Check sheet for the modelled part. Datum: model origin and axes. Units: mm. Face numbers are marked on the shaded views. A direction names the side the tool comes from. Round coordinates to 2 decimals unless told otherwise and drop trailing zeros. Write each loop counter-clockwise with the first axis right and the second up, starting at its lowest first coordinate (ties: lowest second). Pieces come first, ordered by that corner, then holes.
Item 1: Cross-section at D-D on x = 40. Enter the section's corners in (y, z).
Item 2: Cross-section at A-A on y = 15. Enter the section's corners in (x, z).
Item 3: Cross-section at B-B on y = -15.5. Enter the section's corners in (x, z), plus the area to 3 significant figures.
Item 4: Cross-section at C-C on z = 17. Enter the section's corners in (x, y), plus the area to 3 significant figures.
Item 5: Go/stop test with flat-tipped pins: pin 1 Ø8 at (x, y) = (12, 8.5) entering from +Z; pin 2 Ø1.5 at (y, z) = (4, -26) entering from -X; pin 3 Ø8 at (x, y) = (-34, 4.5) entering from -Z. Record where each tip stops, or that it passes through.
Item 6: Material ranges on line 1 (Z direction, x = -13.5, y = 5); line 2 (Z direction, x = 12, y = 14); line 3 (X direction, y = 9, z = -22), recorded low to high.
Item 7: Tool access check on the marked faces 1 and 2. Record the directions out of +Z, -Z, +X, -X, +Y, -Y that give a thin tool (end or side, any length) a straight path to the whole face; none if there is none.
Item 8: Release check for a two-part mould opening along Z. For the marked faces 3, 4 and 5 record: +Z half, -Z half, draft (parallel to the pull), parting line (faces both ways), or undercut.
from build123d import *

# Parameters (mm, degrees)
F1_DEPTH = 20
F2_DEPTH = 20


with BuildPart() as f1:
    # F0 (on Front) → F1 (new body, symmetric)
    with BuildSketch(Plane.XZ):
        Polygon((16.16565, -44.080839), (34.79936, -31.519093), (45.460955, -11.736702), (45.707994, 10.734426), (35.483882, 30.746426), (17.130841, 43.714791), (-5.14667, 46.668624), (-26.245141, 38.931237), (-41.331166, 22.275173), (-46.948719, 0.516136), (-41.810887, -21.361142), (-27.094684, -38.34484), (-6.171415, -46.544197), align=None)
        Polygon((21.260118, -15.324641), (11.703184, -23.449365), (-0.534809, -26.202123), (-12.650283, -22.952289), (-21.86773, -14.444363), (-26.075544, -2.627408), (-24.309764, 9.791456), (-16.974911, 19.967214), (-5.75131, 25.568725), (6.789846, 25.312748), (17.775531, 19.257927), (24.689056, 8.791346), (25.946615, -3.689226), align=None, mode=Mode.SUBTRACT)
    extrude(amount=F1_DEPTH, both=True)

    # F0 (on Front) → F2 (join)
    with BuildSketch(Plane.XZ):
        Polygon((-0.534809, -26.202123), (11.703184, -23.449365), (21.260118, -15.324641), (25.946615, -3.689226), (24.689056, 8.791346), (17.775531, 19.257927), (6.789846, 25.312748), (-5.75131, 25.568725), (-16.974911, 19.967214), (-24.309764, 9.791456), (-26.075544, -2.627408), (-21.86773, -14.444363), (-12.650283, -22.952289), align=None)
    extrude(amount=F2_DEPTH)


solid = f1.part
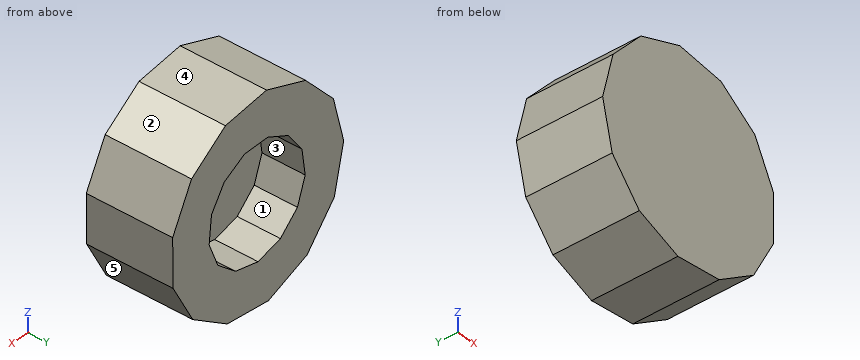
Response values:
1. outline: (-20, -21.87) - (20, -21.87) - (20, 21.91) - (-20, 21.91) - close
2. outline: (-46.95, 0.52) - (-41.81, -21.36) - (-27.09, -38.34) - (-6.17, -46.54) - (16.17, -44.08) - (34.8, -31.52) - (45.46, -11.74) - (45.71, 10.73) - (35.48, 30.75) - (17.13, 43.71) - (-5.15, 46.67) - (-26.25, 38.93) - (-41.33, 22.28) - close; hole (-26.08, -2.63) - (-21.87, -14.44) - (-12.65, -22.95) - (-0.53, -26.2) - (11.7, -23.45) - (21.26, -15.32) - (25.95, -3.69) - (24.69, 8.79) - (17.78, 19.26) - (6.79, 25.31) - (-5.75, 25.57) - (-16.97, 19.97) - (-24.31, 9.79) - close
3. outline: (-46.95, 0.52) - (-41.81, -21.36) - (-27.09, -38.34) - (-6.17, -46.54) - (16.17, -44.08) - (34.8, -31.52) - (45.46, -11.74) - (45.71, 10.73) - (35.48, 30.75) - (17.13, 43.71) - (-5.15, 46.67) - (-26.25, 38.93) - (-41.33, 22.28) - close
3. area: 6,660 mm2
4. outline: (-42.69, -20) - (42.51, -20) - (42.51, 20) - (19.27, 20) - (19.27, 0) - (-19.11, 0) - (-19.11, 20) - (-42.69, 20) - close
4. area: 2,640 mm2
5. pin 1: stops at z = 44.93
5. pin 2: stops at x = -38.44
5. pin 3: stops at z = -34.99
6. line 1: z = -43.67 to -22.17, 21.7 to 43.61
6. line 2: z = -44.54 to -23.2, 22.44 to 44.4
6. line 3: x = -41.26 to -13.68, 13.41 to 39.93
7. face 1: +Y
7. face 2: +Z, +X, +Y, -Y
8. face 3: undercut
8. face 4: +Z half
8. face 5: -Z half
